from build123d import *

# Parameters (mm, degrees)
SKETCH_1_W          = 34
SKETCH_1_H          = 40
SKETCH_1_R          = 2.25
EXTRUDE_1_DEPTH     = 5
SKETCH_2_W          = 34
SKETCH_2_H          = 4
EXTRUDE_2_DEPTH     = 20
SKETCH_3_W          = 34
SKETCH_3_H          = 40
EXTRUDE_3_DEPTH     = 5
SKETCH_4_R          = 1.7
CUT_EXTRUDE_1_DEPTH = 5
FILLET_1_R          = 1.5


with BuildPart() as part:
    # 草图1 → 凸台-拉伸1 (new body)
    with BuildSketch(Plane(origin=(0, 0, 0), x_dir=(0, 0, -1), z_dir=(1, 0, 0))):
        with Locations((17, 20)):
            Rectangle(SKETCH_1_W, SKETCH_1_H)
        with Locations((8, 32)):
            Circle(SKETCH_1_R, mode=Mode.SUBTRACT)
        with Locations((8, 6)):
            Circle(SKETCH_1_R, mode=Mode.SUBTRACT)
        with Locations((26, 32)):
            Circle(SKETCH_1_R, mode=Mode.SUBTRACT)
        with Locations((26, 6)):
            Circle(SKETCH_1_R, mode=Mode.SUBTRACT)
    extrude(amount=EXTRUDE_1_DEPTH)

    # 草图2 → 凸台-拉伸2 (add)
    with BuildSketch(Plane(origin=(5, 0, 0), x_dir=(0, 0, -1), z_dir=(1, 0, 0))):
        with Locations((17, 38)):
            Rectangle(SKETCH_2_W, SKETCH_2_H)
    extrude(amount=EXTRUDE_2_DEPTH)

    # 草图3 → 凸台-拉伸3 (add)
    with BuildSketch(Plane(origin=(25, 0, 0), x_dir=(0, 0, -1), z_dir=(1, 0, 0))):
        with Locations((17, 20)):
            Rectangle(SKETCH_3_W, SKETCH_3_H)
    extrude(amount=EXTRUDE_3_DEPTH)

    # 草图4 → 切除-拉伸1 (cut)
    with BuildSketch(Plane(origin=(30, 0, 0), x_dir=(0, 0, -1), z_dir=(1, 0, 0))):
        with Locations((11.5, 28)):
            Circle(SKETCH_4_R)
        with Locations((22.5, 28)):
            Circle(SKETCH_4_R)
        with Locations((11.5, 9)):
            Circle(SKETCH_4_R)
        with Locations((22.5, 9)):
            Circle(SKETCH_4_R)
    extrude(amount=-CUT_EXTRUDE_1_DEPTH, mode=Mode.SUBTRACT)

    # 圆角1
    fillet_1_edges = [part.edges().sort_by_distance(p)[0] for p in [
        (25, 0, -17),
        (30, 0, -17),
        (30, 40, -17),
        (0, 40, -17),
        (0, 0, -17),
        (5, 0, -17),
    ]]
    fillet(fillet_1_edges, radius=FILLET_1_R)


solid = part.part
Part model, mm, in its own coordinate system. A direction names the side the tool comes from. Coordinates: 2 decimals unless noted, no trailing zeros. Order: outer loops, then holes, each group sorted by start corner. A loop starts at its lowest first (then second) coordinate and runs counter-clockwise, first axis right, second up. Notation, with made-up numbers: (8.5, 4.5) - (46.5, 4.5) arc R20 ccw to (46.5, 30.5) - close; hole circle Ø8 at (10.25, 3). An arc over 180 degrees is marked (long way). Use CSV: the item, a comma, the result in double quotes.
Item 1: 3-axis set-ups, long thin cutter, end or side, ignore diameter. For faces 1 (the face through (15, 36, -17)), 2 (the face through (2.465, 6.099, -5.752)), 3 (the face through (27.535, 29.433, -12.414)), 4 (the face through (0.45, 39.57, -17.24)), 5 (the face through (29.55, 0.43, -17.24)): which of +Z, -Z, +X, -X, +Y, -Y reach the whole face in a straight line?
Solved:
face 1,"+Z, -Z, -Y"
face 2,"-X"
face 3,"+X"
face 4,"+Z, -Z, -X, +Y"
face 5,"+Z, -Z, +X, -Y"
Item 2: Drop flat-ended pins along their axis: P1, Ø2.5, axis at y = 9, z = -22.5, coming from the +X side; P2, Ø10, axis at x = 17, z = -10, coming from the -Y side. Give the stop position or say it passes through.
Solved:
P1,"stops at x = 5"
P2,"stops at y = 36"
Item 3: Saw through at A-A on y = 9. Give the cut face in (x, z), and give its area (3 significant figures).
Solved:
outline,"(0, -34) - (5, -34) - (5, 0) - (0, 0) - close; (25, -34) - (30, -34) - (30, -24.2) - (25, -24.2) - close; (25, -20.8) - (30, -20.8) - (30, -13.2) - (25, -13.2) - close; (25, -9.8) - (30, -9.8) - (30, 0) - (25, 0) - close"
area,"306 mm²"
Item 4: Saw through at D-D on z = -11.5. Give the cut face in (x, y), and give its area (3 significant figures).
Solved:
outline,"(0, 1.5) arc R1.5 ccw to (1.5, 0) - (3.5, 0) arc R1.5 ccw to (5, 1.5) - (5, 36) - (25, 36) - (25, 29.7) - (30, 29.7) - (30, 38.5) arc R1.5 ccw to (28.5, 40) - (1.5, 40) arc R1.5 ccw to (0, 38.5) - close; (25, 1.5) arc R1.5 ccw to (26.5, 0) - (28.5, 0) arc R1.5 ccw to (30, 1.5) - (30, 7.3) - (25, 7.3) - close; (25, 10.7) - (30, 10.7) - (30, 26.3) - (25, 26.3) - close"
area,"443 mm²"
Item 5: Probe probe 1 along Y at (x, z) = (1.5, -26); probe 2 along X at (y, z) = (31, -11); probe 3 along Z at (x, y) = (4.5, 8). List the from-to ranges inside material, lowest first.
Solved:
probe 1,"y = 0 to 3.75, 8.25 to 29.75, 34.25 to 40"
probe 2,"x = 0 to 5, 25 to 30"
probe 3,"z = -34 to -27.03, -24.97 to -9.03, -6.97 to 0"
Item 6: Saw through at B-B on z = -26. Give the cut face in (x, y), and give its area (3 significant figures).
Solved:
outline,"(0, 1.5) arc R1.5 ccw to (1.5, 0) - (3.5, 0) arc R1.5 ccw to (5, 1.5) - (5, 3.75) - (0, 3.75) - close; (0, 8.25) - (5, 8.25) - (5, 29.75) - (0, 29.75) - close; (0, 34.25) - (5, 34.25) - (5, 36) - (25, 36) - (25, 1.5) arc R1.5 ccw to (26.5, 0) - (28.5, 0) arc R1.5 ccw to (30, 1.5) - (30, 38.5) arc R1.5 ccw to (28.5, 40) - (1.5, 40) arc R1.5 ccw to (0, 38.5) - close"
area,"432 mm²"
Item 7: Saw through at C-C on x = 3. Give the cut face in (y, z).
Solved:
outline,"(0, -34) - (40, -34) - (40, 0) - (0, 0) - close; hole circle Ø4.5 at (6, -26); hole circle Ø4.5 at (6, -8); hole circle Ø4.5 at (32, -26); hole circle Ø4.5 at (32, -8)"
Item 8: Mould opens along Z. For faces 6 (the face through (4.8, 24.2, 0)), 7 (the face through (4.55, 0.43, -17.24)), 8 (the face through (2.465, 6.676, -28.146)) say: +Z half, -Z half, draft (parallel to the pull), parting line (faces both ways), or undercut.
Solved:
face 6,"+Z half"
face 7,"draft"
face 8,"undercut"
